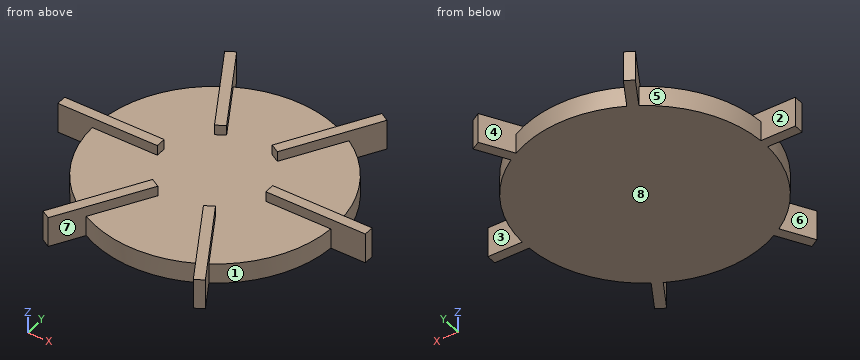
from build123d import *

# Parameters (mm, degrees)
CIRCLE_R         = 60
EXTRUDE067_DEPTH = 10
ARRAY019_W       = 5
ARRAY019_H       = 50
EXTRUDE066_DEPTH = 15


with BuildPart() as extrude093:
    # Circle → Extrude067 (new body)
    with BuildSketch(Plane.XY):
        Circle(CIRCLE_R)
    extrude(amount=EXTRUDE067_DEPTH)


with BuildPart() as fusion045:
    # Array019 → Extrude066 (new body)
    with BuildSketch(Plane(origin=(52.270737, 0, 0), x_dir=(0, 1, 0), z_dir=(0, 0, 1))):
        Rectangle(ARRAY019_W, ARRAY019_H)
        Polygon((22.367151, 36.470305), (65.668421, 11.470305), (68.168421, 15.800432), (24.867151, 40.800432), align=None)
        Polygon((24.867151, 63.741042), (68.168421, 88.741042), (65.668421, 93.071169), (22.367151, 68.071169), align=None)
        with Locations((0, 104.541473)):
            Rectangle(ARRAY019_W, ARRAY019_H)
        Polygon((-22.367151, 68.071169), (-65.668421, 93.071169), (-68.168421, 88.741042), (-24.867151, 63.741042), align=None)
        Polygon((-24.867151, 40.800432), (-68.168421, 15.800432), (-65.668421, 11.470305), (-22.367151, 36.470305), align=None)
    extrude(amount=EXTRUDE066_DEPTH)

    # Fusion045: union Extrude093
    add(extrude093.part)


with BuildPart() as fusion045_1:
    # Fusion045 placement: moved
    add(fusion045.part.moved(Location((150, -307.572449, 20))))


solid = fusion045_1.part
The model under review builds one solid part; all positions refer to its coordinate system, in mm. Face numbers are marked on the shaded views. A direction names the side the tool comes from. Round coordinates to 2 decimals unless told otherwise and drop trailing zeros. Write each loop counter-clockwise with the first axis right and the second up, starting at its lowest first coordinate (ties: lowest second). Pieces come first, ordered by that corner, then holes. Notation, with made-up numbers: (45.5, -6) -> (57.5, -6) arc R16 cw to (57.5, 25) -> close; hole circle Ø2 at (58.5, 88.25). An arc over 180 degrees is marked (long way). Answer as a JSON object with one key per item and string values.
1. Machinability: for the marked faces 1, 2, 3, 4 and 5, which of the approach directions +Z, -Z, +X, -X, +Y, -Y give a long, thin tool a straight path to every point of the face, cutting with its end or side? Answer none if there is none.
Results found:
{"face 1": "+Z, -Z, +X", "face 2": "+Z, -X", "face 3": "+Z, +X", "face 4": "+Z, +Y", "face 5": "+Z, -Z, -X"}
2. We need section A-A on z = 21.75. State the section outline as (x, y) points, and give its area (3 significant figures).
Results found:
{"outline": "(72.73, -310.07) -> (90.05, -310.07) arc R60 ccw to (117.86, -358.24) -> (109.2, -373.24) -> (113.53, -375.74) -> (122.19, -360.74) arc R60 ccw to (177.81, -360.74) -> (186.47, -375.74) -> (190.8, -373.24) -> (182.14, -358.24) arc R60 ccw to (209.95, -310.07) -> (227.27, -310.07) -> (227.27, -305.07) -> (209.95, -305.07) arc R60 ccw to (182.14, -256.91) -> (190.8, -241.9) -> (186.47, -239.4) -> (177.81, -254.41) arc R60 ccw to (122.19, -254.41) -> (113.53, -239.4) -> (109.2, -241.9) -> (117.86, -256.91) arc R60 ccw to (90.05, -305.07) -> (72.73, -305.07) -> close", "area": "11,800 mm^2"}
3. We need section D-D on x = 208. State the section outline as (y, z) points, and give its area (3 significant figures).
Results found:
{"outline": "(-322.93, 20) -> (-292.21, 20) -> (-292.21, 30) -> (-305.07, 30) -> (-305.07, 35) -> (-310.07, 35) -> (-310.07, 30) -> (-322.93, 30) -> close", "area": "332 mm^2"}
4. The part is to be moulded in two halves that separate along X. For the marked faces 6, 7 and 8, say which applies: pulls with the +X half, pulls with the -X half, needs draft (parallel to the pull), parting line crosses it, or undercut.
Results found:
{"face 6": "pulls with the -X half", "face 7": "undercut", "face 8": "needs draft"}
5. We need section B-B on y = -362.5. State the section outline as (x, z) points, and give its area (3 significant figures).
Results found:
{"outline": "(115.4, 20) -> (121.17, 20) -> (121.17, 35) -> (115.4, 35) -> close; (125.86, 20) -> (174.14, 20) -> (174.14, 30) -> (125.86, 30) -> close; (178.83, 20) -> (184.6, 20) -> (184.6, 35) -> (178.83, 35) -> close", "area": "656 mm^2"}
6. Clearance check with flat-ended pins moving along their axes: pin 1 (4 mm diameter, centred on x = 100, z = 27, fed in from -Y); pin 2 (3 mm diameter, centred on y = -296, z = 23, fed in from -X); pin 3 (3 mm diameter, centred on x = 147, z = 27.5, fed in from -Y). State where each tip first meets the part, or that it passes through.
Results found:
{"pin 1": "stops at y = -343.57", "pin 2": "stops at x = 90.85", "pin 3": "stops at y = -367.55"}
7. We need section C-C on y = -307. State the section outline as (x, z) points, and give its area (3 significant figures).
Results found:
{"outline": "(72.73, 20) -> (227.27, 20) -> (227.27, 35) -> (177.27, 35) -> (177.27, 30) -> (122.73, 30) -> (122.73, 35) -> (72.73, 35) -> close", "area": "2,050 mm^2"}
8. To check wall thickness, follow line 1 along X through (y, z) = (-252.5, 27.75); line 2 along X through (y, z) = (-254, 24.75); line 3 along Y through (x, z) = (211, 30.5). State the ranges of each line that lie inside material, in increasing order.
Results found:
{"line 1": "x = 115.32 to 121.09, 126.19 to 173.81, 178.91 to 184.68", "line 2": "x = 116.18 to 121.96, 122.98 to 177.02, 178.04 to 183.82", "line 3": "y = -310.07 to -305.07"}
